For this review, take the finished solid that the model builds, in its own axes (mm). A direction names the side the tool comes from. Round coordinates to 2 decimals unless told otherwise and drop trailing zeros. Order: outer loops, then holes, each group sorted by start corner. A loop starts at its lowest first (then second) coordinate and runs counter-clockwise, first axis right, second up. Notation, with made-up numbers: (20, -35) - (52, -35) arc R30 ccw to (52, -4) - close; hole circle Ø10 at (-28, 9). An arc over 180 degrees is marked (long way). Write each question's results on one line, items separated by ' | '. Start each with the question number.
(1) Insertion check: pin 1 Ø12 at (x, z) = (25, -10.5) entering from -Y; pin 2 Ø17.5 at (y, z) = (23, -41.5) entering from -X; pin 3 Ø13 at (y, z) = (12.5, 8) entering from -X; pin 4 Ø1.5 at (y, z) = (15.5, -38.5) entering from +X. Each pin has a flat end and moves straight along its axis. Give the tip position at first contact, or say it passes through.
(2) Take a section at B-B, the plane x = -30. Give the boundary of the cut face in (y, z).
(3) Draft analysis for pull direction X (two halves, no side actions). For faces 1 (the flat face through (-9, 25, 45.456)), 2 (the flat face through (-8.94, 12.39, 9.07)), 3 (the cylindrical face through (29.51, 3.46, -2.71)), state which applies: pulls with the +X half, pulls with the -X half, needs draft (parallel to the pull), parting line crosses it, or undercut.
(4) For L1, parallel to Y at x = -40, z = 18; L2, parallel to X at y = 10.5, z = 12.5; L3, parallel to X at y = 14.5, z = 8.5, list the stretches that pass through material, from the lowest coordinate up. Write a range as from..to.
(5) Take a section at C-C, the plane z = 17. Give the number of separate pieces and of enclosed holes in the cut face, plus the area to 3 significant figures.
(6) Take a section at A-A, the plane x = -44. Give the boundary of the cut face in (y, z).
(7) For faces 4 (the flat face through (-9, 25, -49.544)), 5 (the flat face through (-39, 21, -27.544)), 6 (the flat face through (-32.697, 12, -2)), 7 (the flat face through (-35, 21, 23.456)), 8 (the flat face through (-6.724, 13.184, -1.919)), list the 3-axis set-ups (+Z, -Z, +X, -X, +Y, -Y) from which the entire face can be reached by the end or side of a thin tool; tool diameter is ignored.
(8) Take a section at D-D, the plane y = 47. Give the boundary of the cut face in (x, z), plus the area to 3 significant figures.
```python
from build123d import *

# Parameters (mm, degrees)
SKETCH1_W           = 95
SKETCH1_H           = 95
BOSS_EXTRUDE1_DEPTH = 50
CUT_EXTRUDE1_DEPTH  = 100
SKETCH3_R           = 9.5
CUT_EXTRUDE2_DEPTH  = 45
CUT_EXTRUDE4_DEPTH  = 45
CUT_EXTRUDE5_DEPTH  = 45
CUT_EXTRUDE6_DEPTH  = 45
CUT_EXTRUDE7_DEPTH  = 45
SKETCH9_R           = 9.5
CUT_EXTRUDE9_DEPTH  = 45
SKETCH11_R          = 9.5
CUT_EXTRUDE10_DEPTH = 45
SKETCH12_W          = 31.985759797
SKETCH12_H          = 95
BOSS_EXTRUDE2_DEPTH = 45
CUT_EXTRUDE11_DEPTH = 100
SKETCH14_R          = 9.5
CUT_EXTRUDE12_DEPTH = 100
SKETCH15_R          = 9.5
CUT_EXTRUDE13_DEPTH = 100
SKETCH16_R          = 9.5
CUT_EXTRUDE14_DEPTH = 100
FILLET2_R           = 4
SKETCH17_W          = 34
SKETCH17_H          = 34
CUT_EXTRUDE16_DEPTH = 22
SKETCH19_W          = 34
SKETCH19_H          = 34
CUT_EXTRUDE17_DEPTH = 22
SKETCH20_W          = 12.5
SKETCH20_H          = 16.5
CUT_EXTRUDE18_DEPTH = 60
CUT_EXTRUDE19_DEPTH = 60


with BuildPart() as part:
    # Sketch1 → Boss-Extrude1 (new body)
    with BuildSketch(Plane(origin=(0, 0, 0), x_dir=(1, 0, 0), z_dir=(0, 1, 0))):
        with Locations((-8.446550514, 2.043801884)):
            Rectangle(SKETCH1_W, SKETCH1_H)
    extrude(amount=BOSS_EXTRUDE1_DEPTH)

    # Sketch2 → Cut-Extrude1 (cut)
    with BuildSketch(Plane.XY.offset(45.456198116)):
        Polygon((39.053449486, 0), (36.353449486, 50), (39.053449486, 50), align=None)
    extrude(amount=-CUT_EXTRUDE1_DEPTH, mode=Mode.SUBTRACT)

    # Sketch3 → Cut-Extrude2 (cut)
    with BuildSketch(Plane(origin=(38.939900735, 2.10275464, 0), x_dir=(0, 0, -1), z_dir=(0.998545181, 0.05392144, 0))):
        with Locations((2.043801884, 13.394181776)):
            Circle(SKETCH3_R)
    extrude(amount=-CUT_EXTRUDE2_DEPTH, mode=Mode.SUBTRACT)

    # Sketch5 → Cut-Extrude4 (cut)
    with BuildSketch(Plane(origin=(0, 50, 0), x_dir=(1, 0, 0), z_dir=(0, 1, 0))):
        Polygon((39.053449486, 49.543801884), (39.053449486, 29.543801884), (19.053449486, 49.543801884), align=None)
        Polygon((39.053449486, -45.456198116), (39.053449486, -25.456198116), (19.053449486, -45.456198116), align=None)
    extrude(amount=-CUT_EXTRUDE4_DEPTH, mode=Mode.SUBTRACT)

    # Sketch6 → Cut-Extrude5 (cut)
    with BuildSketch(Plane(origin=(0, 50, 0), x_dir=(1, 0, 0), z_dir=(0, 1, 0))):
        Polygon((19.053449486, -45.456198116), (12.925569587, -39.328318218), (6.797689689, -45.456198116), align=None)
        Polygon((19.053449486, 49.543801884), (12.925569587, 43.415921985), (6.797689689, 49.543801884), align=None)
    extrude(amount=-CUT_EXTRUDE5_DEPTH, mode=Mode.SUBTRACT)

    # Sketch7 → Cut-Extrude6 (cut)
    with BuildSketch(Plane(origin=(-13.201374315, 0, 13.201374315), x_dir=(0.707106781, 0, 0.707106781), z_dir=(-0.707106781, 0, 0.707106781))):
        Polygon((45.615209271, 5), (42.915209271, 50), (45.615209271, 50), align=None)
    extrude(amount=-CUT_EXTRUDE6_DEPTH, mode=Mode.SUBTRACT)

    # Sketch8 → Cut-Extrude7 (cut)
    with BuildSketch(Plane(origin=(-15.245176199, 0, -15.245176199), x_dir=(-0.707106781, 0, 0.707106781), z_dir=(-0.707106781, 0, -0.707106781))):
        Polygon((-48.505581614, 5), (-45.805581614, 50), (-48.505581614, 50), align=None)
    extrude(amount=-CUT_EXTRUDE7_DEPTH, mode=Mode.SUBTRACT)

    # Sketch9 → Cut-Extrude9 (cut)
    with BuildSketch(Plane(origin=(34.386964646, 2.917830706, -34.386964646), x_dir=(-0.708373873, 0.059677836, -0.70331004), z_dir=(0.705837415, 0.059892291, -0.705837415))):
        with Locations((14.526974541, 11.311121921)):
            Circle(SKETCH9_R)
    extrude(amount=-CUT_EXTRUDE9_DEPTH, mode=Mode.SUBTRACT)

    # Sketch11 → Cut-Extrude10 (cut)
    with BuildSketch(Plane(origin=(32.350494057, 2.745030447, 32.350494057), x_dir=(0.70331004, 0.059677836, -0.708373873), z_dir=(0.705837415, 0.059892291, 0.705837415))):
        with Locations((-10.17752107, 12.964151979)):
            Circle(SKETCH11_R)
    extrude(amount=-CUT_EXTRUDE10_DEPTH, mode=Mode.SUBTRACT)

    # Sketch12 → Boss-Extrude2 (add)
    with BuildSketch(Plane(origin=(0, 5, 0), x_dir=(1, 0, 0), z_dir=(0, 1, 0))):
        with Locations((22.790569588, 2.043801884)):
            Rectangle(SKETCH12_W, SKETCH12_H)
    extrude(amount=BOSS_EXTRUDE2_DEPTH)

    # Sketch13 → Cut-Extrude11 (cut)
    with BuildSketch(Plane.XY.offset(45.456198116)):
        Polygon((39.053449486, 0), (29.053449486, 3), (19.053449486, 50), (49.745275601, 50), align=None)
    extrude(amount=-CUT_EXTRUDE11_DEPTH, mode=Mode.SUBTRACT)

    # Sketch14 → Cut-Extrude12 (cut)
    with BuildSketch(Plane(origin=(-5.994632406, -0.32371015, 0), x_dir=(0, 0, -1), z_dir=(0.998545181, 0.05392144, 0))):
        with Locations((2.043801884, 13.394181776)):
            Circle(SKETCH14_R)
    extrude(amount=CUT_EXTRUDE12_DEPTH, mode=Mode.SUBTRACT)

    # Sketch15 → Cut-Extrude13 (cut)
    with BuildSketch(Plane(origin=(0.587810371, 0.049877364, 0.587810371), x_dir=(0.70331004, 0.059677836, -0.708373873), z_dir=(0.705837415, 0.059892291, 0.705837415))):
        with Locations((-10.17752107, 12.964151979)):
            Circle(SKETCH15_R)
    extrude(amount=CUT_EXTRUDE13_DEPTH, mode=Mode.SUBTRACT)

    # Sketch16 → Cut-Extrude14 (cut)
    with BuildSketch(Plane(origin=(2.62428096, 0.222677624, -2.62428096), x_dir=(-0.708373873, 0.059677836, -0.70331004), z_dir=(0.705837415, 0.059892291, -0.705837415))):
        with Locations((14.526974541, 11.311121921)):
            Circle(SKETCH16_R)
    extrude(amount=CUT_EXTRUDE14_DEPTH, mode=Mode.SUBTRACT)

    # Fillet2
    fillet2_edges = [part.edges().sort_by_distance(p)[0] for p in [
        (29.053449486, 3, -2.043801884),
    ]]
    fillet(fillet2_edges, radius=FILLET2_R)

    # Sketch17 → Cut-Extrude16 (cut)
    with BuildSketch(Plane.XY.offset(45.456198116)):
        with Locations((-38.946550514, 17)):
            Rectangle(SKETCH17_W, SKETCH17_H)
    extrude(amount=-CUT_EXTRUDE16_DEPTH, mode=Mode.SUBTRACT)

    # Sketch19 → Cut-Extrude17 (cut)
    with BuildSketch(Plane(origin=(0, 0, -49.543801884), x_dir=(-1, 0, 0), z_dir=(0, 0, -1))):
        with Locations((38.946550514, 17)):
            Rectangle(SKETCH19_W, SKETCH19_H)
    extrude(amount=-CUT_EXTRUDE17_DEPTH, mode=Mode.SUBTRACT)

    # Sketch20 → Cut-Extrude18 (cut)
    with BuildSketch(Plane.XY.offset(23.456198116)):
        with Locations((-38.946550514, 12.25)):
            Rectangle(SKETCH20_W, SKETCH20_H)
    extrude(amount=-CUT_EXTRUDE18_DEPTH, mode=Mode.SUBTRACT)

    # Sketch21 → Cut-Extrude19 (cut)
    with BuildSketch(Plane.XY.offset(23.456198116)):
        Polygon((-55.946550514, 34), (-48.446550514, 0), (-55.946550514, 0), align=None)
    extrude(amount=-CUT_EXTRUDE19_DEPTH, mode=Mode.SUBTRACT)


solid = part.part
```
Results below:
1) pin 1: stops at y = 0 | pin 2: stops at x = -21.95 | pin 3: stops at x = -52.64 | pin 4: stops at x = 6.42
2) outline: (0, -27.54) - (34, -27.54) - (34, -49.54) - (50, -49.54) - (50, 45.46) - (34, 45.46) - (34, 23.46) - (0, 23.46) - close
3) face 1: needs draft | face 2: undercut | face 3: pulls with the +X half
4) L1: y = 0..4, 20.5..50 | L2: x = -50.76..-45.2, -32.7..-12.21, 9.88..27.46 | L3: x = -51.65..-45.2, -32.7..-8.55, 6.3..26.61
5) separate pieces: 1 | enclosed holes: 2 | area: 3,300 mm^2
6) outline: (0, -27.54) - (4, -27.54) - (4, 23.46) - (0, 23.46) - close; (20.5, -27.54) - (34, -27.54) - (34, -49.54) - (50, -49.54) - (50, 45.46) - (34, 45.46) - (34, 23.46) - (20.5, 23.46) - close
7) face 4: -Z, +X, -X, +Y, -Y | face 5: -Z, -X, -Y | face 6: +Z, -Z | face 7: +Z, -X, -Y | face 8: none
8) outline: (-55.95, -49.54) - (19.69, -49.54) - (19.69, 45.46) - (-55.95, 45.46) - close | area: 7,190 mm^2
